```python
from build123d import *

# Parameters (mm, degrees)
SKETCH_R        = 9
SKETCH_R_2      = 4
PAD_DEPTH       = 10
COPYSKETCH001_W = 20
COPYSKETCH001_H = 20
POCKET_DEPTH    = 10.001
FILLET_R        = 10


with BuildPart() as part:
    # Sketch → Pad (new body)
    with BuildSketch(Plane.XZ):
        with BuildLine():
            Line((0, 0), (0, 25))
            Line((0, 25), (-10, 25))
            Line((-10, 25), (-10, 55))
            Line((-10, 55), (0, 55))
            Line((0, 55), (0, 80))
            Line((0, 80), (-10, 80))
            Line((-10, 80), (-10, 110))
            Line((-10, 110), (0, 110))
            Line((0, 110), (0, 125))
            Line((0, 125), (-10.439, 125))
            ThreePointArc((-24.439, 139), (-20.338495, 129.100505), (-10.439, 125))
            Line((-24.439, 139), (-24.439, 151.456))
            ThreePointArc((12.872585, 161.471439), (-9.623992, 170.772207), (-24.439, 151.456))
            ThreePointArc((12.872585, 161.471439), (26.413305, 147.948816), (44.899018, 143))
            Line((44.899018, 143), (230, 143))
            Line((230, 143), (230, 131.156))
            Line((230, 131.156), (240, 131.156))
            Line((240, 131.156), (240, 101.156))
            Line((240, 101.156), (230, 101.156))
            Line((230, 101.156), (230, 61.156))
            Line((230, 61.156), (240, 61.156))
            Line((240, 61.156), (240, 31.156))
            Line((240, 31.156), (230, 31.156))
            Line((230, 31.156), (230, 25))
            ThreePointArc((230, 25), (219.393398, 20.606602), (215, 10))
            Line((215, 10), (211, 10))
            Line((211, 10), (211, 0))
            Line((211, 0), (131, 0))
            Line((131, 0), (131, 10))
            Line((131, 10), (80, 10))
            Line((80, 10), (80, 0))
            Line((80, 0), (0, 0))
        make_face()
        with Locations((15, 25)):
            Circle(SKETCH_R, mode=Mode.SUBTRACT)
        with Locations((-5.055, 150.4)):
            Circle(SKETCH_R_2, mode=Mode.SUBTRACT)
    extrude(amount=PAD_DEPTH)

    # CopySketch001 → Pocket (cut, through all)
    with BuildSketch(Plane.XZ):
        with BuildLine():
            ThreePointArc((74.93, 112.3), (114.93, 72.3), (154.93, 112.3))
            Line((154.93, 112.3), (154.93, 155.12))
            Line((74.93, 155.12), (154.93, 155.12))
            Line((74.93, 112.3), (74.93, 155.12))
        make_face()
        with Locations((114.93, 30)):
            Rectangle(COPYSKETCH001_W, COPYSKETCH001_H)
    extrude(amount=POCKET_DEPTH, mode=Mode.SUBTRACT)

    # Fillet
    fillet_edges = [part.edges().sort_by_distance(p)[0] for p in [
        (154.93, -5, 143),
        (74.93, -5, 143),
    ]]
    fillet(fillet_edges, radius=FILLET_R)


solid = part.part
```
Read the model definition and answer for the solid it produces. Units are mm, in the model's axes. A direction names the side the tool comes from. Give positions to 0.01 mm unless a question says otherwise; leave off trailing zeros. Order: outer loops, then holes, each group sorted by start corner. A loop starts at its lowest first (then second) coordinate and runs counter-clockwise, first axis right, second up. Notation, with made-up numbers: (6.5, 30) -> (61.5, 30) arc R13 cw to (61.5, 46) -> close; hole circle Ø2 at (63, 61). An arc over 180 degrees is marked (long way). One line per item, written item: value. Start each with the question number.
(1) Flat-ended cylindrical pins translate along their axes: P1, Ø5, axis at y = -6, z = 137, coming from the +X side; P2, Ø3, axis at x = 237, y = -6, coming from the +Z side; P3, Ø3, axis at x = 113.5, y = -4.5, coming from the -Z side; P4, Ø1, axis at x = 74.5, z = 106.5, coming from the +Y side. Find the tip coordinate at first contact, or state that the pin passes through.
(2) The part is cut by section B-B (x = 114.93). Determine the outline of the cut face in (y, z), and give its area (3 significant figures).
(3) The part is cut by section A-A (z = 120). Determine the outline of the cut face in (x, y).
(4) A tool of negligible diameter and unlimited length cuts with its end or side. For faces 4 (the flat face through (-10, -5, 95)), 5 (the flat face through (230, -5, 137)), 6 (the flat face through (115, -5, 20)), 7 (the flat face through (-5, -5, 55)), from which of +Z, -Z, +X, -X, +Y, -Y can it reach the whole face along a straight path? Write none if from no direction.
(5) For a pull along Z with two mould halves and no side action, classify faces 1 (the flat face through (0, -5, 67)), 2 (the cylindrical face through (72.08, -5.07, 139.99)), 3 (the flat face through (110, 0, 68)) as released by +Z, released by -Z, zero draft, split by the parting line, or undercut.
(6) The part is cut by section C-C (y = -2). State how many separate pieces and enclosed holes the cut face has, and give its area (3 significant figures).
(7) Straight lines are drawn through the part: L1, parallel to X at y = -2.5, z = 25.5; L2, parallel to X at y = -4.5, z = 38; L3, parallel to X at y = -5, z = 21.5. For each, find the intervals that lie inside material, in ascending order.
Taken from the geometry:
1. P1: x = 230
1. P2: z = 131.16
1. P3: z = 10
1. P4: y = 0
2. outline: (-10, 10) -> (0, 10) -> (0, 20) -> (-10, 20) -> close; (-10, 40) -> (0, 40) -> (0, 72.3) -> (-10, 72.3) -> close
2. area: 423 mm^2
3. outline: (0, -10) -> (74.93, -10) -> (74.93, 0) -> (0, 0) -> close; (154.93, -10) -> (240, -10) -> (240, 0) -> (154.93, 0) -> close
4. face 4: -Z, -X, +Y, -Y
4. face 5: +Z, +X, +Y, -Y
4. face 6: +Y, -Y
4. face 7: -X, +Y, -Y
5. face 1: undercut
5. face 2: released by +Z
5. face 3: zero draft
6. separate pieces: 1
6. enclosed holes: 3
6. area: 29,000 mm^2
7. L1: -10 to 6.01, 23.99 to 104.93, 124.93 to 230
7. L2: -10 to 104.93, 124.93 to 240
7. L3: 0 to 6.71, 23.29 to 104.93, 124.93 to 220.37
